CAD build for the part. Positions are in the model's coordinates, mm. A direction names the side the tool comes from. Give positions to 0.01 mm unless a question says otherwise; leave off trailing zeros. Order: outer loops, then holes, each group sorted by start corner. A loop starts at its lowest first (then second) coordinate and runs counter-clockwise, first axis right, second up.
Item 1: Wall check: L1, parallel to Y at x = 1.8, z = 1.95; L2, parallel to Y at x = -1.05, z = -0.6; L3, parallel to Z at x = -0.9, y = 10.75. Give the ranges that are in metal, low to high.
Item 2: Band-saw the part on B-B on z = 0. Give the cut face in (x, y).
Item 3: Which spindle directions (+Z, -Z, +X, -X, +Y, -Y) get a long thin tool onto all of the face, cutting with end or side? Do faces 4 (the flat face through (0, 1, -0.961)), 5 (the flat face through (0, 0, 2)), 6 (the flat face through (-1.2, 2.4, -1.2)). Say none if no direction does.
Item 4: Band-saw the part on D-D on z = -1.35. Give the cut face in (x, y), plus the area to 3 significant figures.
Item 5: Band-saw the part on C-C on y = 5.75. Give the cut face in (x, z).
Item 6: Two-plate mould, pull along Z, no slides. Class faces 1 (the cylindrical face through (0.607, 1.183, 2.733)), 2 (the flat face through (0, 12.4, 0)), 3 (the flat face through (0, 1.296, 0)): released by +Z, released by -Z, zero draft, split by the parting line, or undercut.
Item 7: Band-saw the part on A-A on x = 0. Give the cut face in (y, z), plus the area to 3 significant figures.
Item 8: Flat gauge pins, fed straight in: P1, Ø2, axis at y = 3.5, z = -0.5, coming from the +X side; P2, Ø1.5, axis at x = 1.5, y = 7, coming from the -Z side; P3, Ø0.6, axis at x = 1, z = 0.5, coming from the -Y side. Where does each tip first touch, or does it go through?
Autodesk Inventor part; units mm, degrees
ref_plane "YZ Plane" through (0, 0, 0) normal (1, 0, 0) x (0, 1, 0)
ref_plane "XZ Plane" through (0, 0, 0) normal (0, 1, 0) x (-1, 0, 0)
ref_plane "XY Plane" through (0, 0, 0) normal (0, 0, 1) x (1, 0, 0)
sketch "Esboço1" plane through (0, 0, 0) normal (0, 1, 0) x (-1, 0, 0)
  circle A0 centre (0, 0) radius 2.8
  dimension "d0" = 5.6
extrude "Extrusão1" add sketch "Esboço1" along normal blind 2.4
sketch "Esboço2" plane through (0, 0, 0) normal (1, 0, 0) x (0, 1, 0)
  line L0 (0, 0.9185) -> (1.2961, 0.9185)
  line L1 (1.2961, 0.9185) -> (1.2961, -0.9611)
  line L2 (1.2961, -0.9611) -> (0, -0.9611)
  line L3 (0, -0.9611) -> (0, 0.9185)
  point P0 (0, 0)
extrude "Extrusão2" cut sketch "Esboço2" along normal through all both and the other way through all
sketch "Esboço3" plane through (0, 2.4, 0) normal (0, 1, 0) x (1, 0, 0)
  circle A0 centre (0, 0) radius 2.8
  circle A1 centre (0, 0) radius 1.5
  dimension "d5" = 3
extrude "Extrusão3" add sketch "Esboço3" along normal blind 10 contours A1
thread "Rosca1"
properties part number "AA-Parafuso-M3-30"
The answers:
1. L1: y = 0 to 2.4
1. L2: y = 1.3 to 12.4
1. L3: z = -1.2 to 1.2
2. outline: (-2.8, 1.3) - (2.8, 1.3) - (2.8, 2.4) - (1.5, 2.4) - (1.5, 12.4) - (-1.5, 12.4) - (-1.5, 2.4) - (-2.8, 2.4) - close
3. face 4: +X, -X, -Y
3. face 5: +Z, -Z, +X, -X, -Y
3. face 6: +Y
4. outline: (-2.45, 0) - (2.45, 0) - (2.45, 2.4) - (0.65, 2.4) - (0.65, 12.4) - (-0.65, 12.4) - (-0.65, 2.4) - (-2.45, 2.4) - close
4. area: 24.9 mm2
5. outline: circle Ø3 at (0, 0)
6. face 1: split by the parting line
6. face 2: zero draft
6. face 3: undercut
7. outline: (0, -2.8) - (2.4, -2.8) - (2.4, -1.5) - (12.4, -1.5) - (12.4, 1.5) - (2.4, 1.5) - (2.4, 2.8) - (0, 2.8) - (0, 0.92) - (1.3, 0.92) - (1.3, -0.96) - (0, -0.96) - close
7. area: 41.0 mm2
8. P1: stops at x = 1.5
8. P2: stops at z = -1.3
8. P3: stops at y = 1.3
